Read the model definition and answer for the solid it produces. Units are mm, in the model's axes. Face numbers are marked on the shaded views. A direction names the side the tool comes from. Round coordinates to 2 decimals unless told otherwise and drop trailing zeros. Answer as CSV lines item,"result".
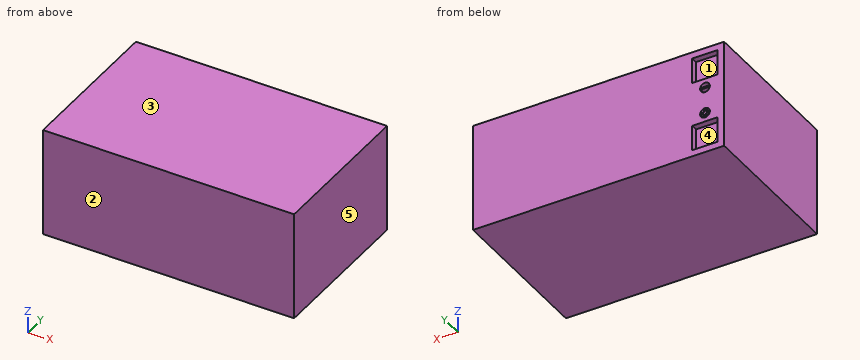
```python
from build123d import *

# Parameters (mm, degrees)
SKETCH1_W           = 150.114
SKETCH1_H           = 64.77
BOSS_EXTRUDE1_DEPTH = 93.472
SKETCH2_R           = 2.91386686
SKETCH2_W           = 15.24
SKETCH2_H           = 15.24
CUT_EXTRUDE1_DEPTH  = 3.81


with BuildPart() as part:
    # Sketch1 → Boss-Extrude1 (new body)
    with BuildSketch(Plane(origin=(0, 0, 0), x_dir=(1, 0, 0), z_dir=(0, 1, 0))):
        with Locations((3.604380952, 5.860142857)):
            Rectangle(SKETCH1_W, SKETCH1_H)
    extrude(amount=BOSS_EXTRUDE1_DEPTH)

    # Sketch2 → Cut-Extrude1 (cut)
    # profile 1 of 4: a face of its own
    with BuildSketch(Plane(origin=(0, 93.472, 0), x_dir=(1, 0, 0), z_dir=(0, 1, 0))):
        with Locations(Location((-60.022619048, -2.026557143, 0), (0, 0, 270))):
            Circle(SKETCH2_R)
        Polygon((-60.022619048, -1.518557143), (-57.482619048, -1.518557143), (-57.482619048, -2.534557143), (-62.562619048, -2.534557143), (-62.562619048, -1.518557143), align=None, mode=Mode.SUBTRACT)
    # profile 2 of 4: a face of its own
    with BuildSketch(Plane(origin=(0, 93.472, 0), x_dir=(1, 0, 0), z_dir=(0, 1, 0))):
        with Locations(Location((-60.022619048, 13.746842857, 0), (0, 0, 270))):
            Circle(SKETCH2_R)
        Polygon((-57.482619048, 13.238842857), (-57.482619048, 14.254842857), (-59.515974161, 14.254842857), (-59.515974161, 16.286842857), (-60.531974161, 16.286842857), (-60.531974161, 14.254842857), (-62.562619048, 14.254842857), (-62.562619048, 13.238842857), (-60.531974161, 13.238842857), (-60.531974161, 11.206842857), (-59.515974161, 11.206842857), (-59.515974161, 13.238842857), align=None, mode=Mode.SUBTRACT)
    # profile 3 of 4: a face of its own
    with BuildSketch(Plane(origin=(0, 93.472, 0), x_dir=(1, 0, 0), z_dir=(0, 1, 0))):
        with Locations((-60.022619048, -15.094857143)):
            Rectangle(SKETCH2_W, SKETCH2_H)
    # profile 4 of 4: a face of its own
    with BuildSketch(Plane(origin=(0, 93.472, 0), x_dir=(1, 0, 0), z_dir=(0, 1, 0))):
        with Locations((-60.022619048, 26.815142857)):
            Rectangle(SKETCH2_W, SKETCH2_H)
    extrude(amount=-CUT_EXTRUDE1_DEPTH, mode=Mode.SUBTRACT)


solid = part.part
```
1) Find the intervals of material crossed by line 1 (Y direction, x = -64, z = -27.5), in increasing order.
Entries:
line 1,"y = 0 to 89.66"
2) The mould has two halves that part along Z. Classify the marked faces 1, 2 and 3: pulls with the +Z half, pulls with the -Z half, needs draft (parallel to the pull), parting line crosses it, or undercut.
Entries:
face 1,"undercut"
face 2,"needs draft"
face 3,"pulls with the +Z half"
3) A tool of negligible diameter and unlimited length cuts with its end or side. For the marked faces 4 and 5, from which of +Z, -Z, +X, -X, +Y, -Y can it reach the whole face along a straight path? Write none if from no direction.
Entries:
face 4,"+Y"
face 5,"+Z, -Z, +X, +Y, -Y"
